from build123d import *

# Parameters (mm, degrees)
SKETCH1_W           = 157.1625
SKETCH1_H           = 96.8375
SKETCH1_R           = 1.5875
SKETCH1_R_2         = 1.27
SKETCH1_R_3         = 3.0861
SKETCH1_W_2         = 2.032
SKETCH1_H_2         = 74.295
BOSS_EXTRUDE1_DEPTH = 2.54


with BuildPart() as part:
    # Sketch1 → Boss-Extrude1 (new body)
    with BuildSketch(Plane(origin=(0, 0, 0), x_dir=(1, 0, 0), z_dir=(0, 1, 0))):
        Rectangle(SKETCH1_W, SKETCH1_H)
        with Locations((-66.51625, 34.44875)):
            Circle(SKETCH1_R, mode=Mode.SUBTRACT)
        with Locations((-61.43625, -17.62125)):
            Circle(SKETCH1_R, mode=Mode.SUBTRACT)
        with Locations((-33.49625, -17.62125)):
            Circle(SKETCH1_R, mode=Mode.SUBTRACT)
        with Locations((-18.25625, 33.17875)):
            Circle(SKETCH1_R, mode=Mode.SUBTRACT)
        with Locations((57.56275, 40.32885)):
            Circle(SKETCH1_R_2, mode=Mode.SUBTRACT)
        with Locations((39.08425, 40.35425)):
            Circle(SKETCH1_R_2, mode=Mode.SUBTRACT)
        with Locations((20.60575, 40.35425)):
            Circle(SKETCH1_R_2, mode=Mode.SUBTRACT)
        with Locations((57.56275, -40.29075)):
            Circle(SKETCH1_R_2, mode=Mode.SUBTRACT)
        with Locations((39.08425, -40.29075)):
            Circle(SKETCH1_R_2, mode=Mode.SUBTRACT)
        with Locations((20.60575, -40.29075)):
            Circle(SKETCH1_R_2, mode=Mode.SUBTRACT)
        with Locations((0, 23.01875)):
            Circle(SKETCH1_R_3, mode=Mode.SUBTRACT)
        with Locations((20.73275, 0.03175)):
            Rectangle(SKETCH1_W_2, SKETCH1_H_2, mode=Mode.SUBTRACT)
        with Locations((39.21125, 0.03175)):
            Rectangle(SKETCH1_W_2, SKETCH1_H_2, mode=Mode.SUBTRACT)
        with Locations((57.68975, 0.03175)):
            Rectangle(SKETCH1_W_2, SKETCH1_H_2, mode=Mode.SUBTRACT)
    extrude(amount=BOSS_EXTRUDE1_DEPTH)


solid = part.part
CAD build for the part. Positions are in the model's coordinates, mm. Round coordinates to 2 decimals unless told otherwise and drop trailing zeros. Order: outer loops, then holes, each group sorted by start corner. A loop starts at its lowest first (then second) coordinate and runs counter-clockwise, first axis right, second up. Notation, with made-up numbers: (14, -28) - (60, -28) arc R24 ccw to (60, 2) - close; hole circle Ø10 at (80, 84.5). An arc over 180 degrees is marked (long way). Return JSON: item names as keys, results as strings.
(1) Pull direction X, two halves, no side cores. Call faces 1 (the face through (-1, 2.54, -1)), 2 (the face through (-2.45, 1.25, -21.14)): +X half, -X half, draft (parallel to the pull), parting line (faces both ways), or undercut.
Answer key:
{"face 1": "draft", "face 2": "undercut"}
(2) Cut at B-B (z = -29). Give the cut face in (x, y).
Answer key:
{"outline": "(-78.58, 0) - (19.72, 0) - (19.72, 2.54) - (-78.58, 2.54) - close; (21.75, 0) - (38.2, 0) - (38.2, 2.54) - (21.75, 2.54) - close; (40.23, 0) - (56.67, 0) - (56.67, 2.54) - (40.23, 2.54) - close; (58.71, 0) - (78.58, 0) - (78.58, 2.54) - (58.71, 2.54) - close"}
(3) Pin check, flat tip, straight feed: pin 1 Ø1.5 at (x, z) = (57.56, 40.29) entering from +Y. Stop position of the tip, or through.
Answer key:
{"pin 1": "passes through"}
(4) Cut at C-C (y = 1.6). State how many separate pieces and enclosed holes the cut face has, then the cut area to 3 significant figures.
Answer key:
{"separate pieces": "1", "enclosed holes": "14", "area": "14,700 mm^2"}
(5) Cut at A-A (x = 0). Give the cut face in (y, z), then the cut area to 3 significant figures.
Answer key:
{"outline": "(0, -48.42) - (2.54, -48.42) - (2.54, -26.1) - (0, -26.1) - close; (0, -19.93) - (2.54, -19.93) - (2.54, 48.42) - (0, 48.42) - close", "area": "230 mm^2"}
(6) Wall check: probe 1 along X at (y, z) = (2.3, 23); probe 2 along Z at (x, y) = (21.5, 2.3); probe 3 along X at (y, z) = (2.2, -39.5) (1 decimal). Give the ranges that are in metal, low to high. Write a range as from..to.
Answer key:
{"probe 1": "x = -78.58..19.72, 21.75..38.2, 40.23..56.67, 58.71..78.58", "probe 2": "z = -48.42..-41.26, -39.45..-37.18, 37.12..39.39, 41.19..48.42", "probe 3": "x = -78.6..19.7, 21.5..38.1, 40..56.6, 58.5..78.6"}
